Design review of the part built by this model. Coordinates are the model's own, in mm. A direction names the side the tool comes from. Round coordinates to 2 decimals unless told otherwise and drop trailing zeros. Order: outer loops, then holes, each group sorted by start corner. A loop starts at its lowest first (then second) coordinate and runs counter-clockwise, first axis right, second up. Notation, with made-up numbers: (74, 59.5) - (124, 59.5) arc R9 cw to (124, 67.5) - close; hole circle Ø9 at (23.5, 20). An arc over 180 degrees is marked (long way). Write item = value, one per line.
from build123d import *

# Parameters (mm, degrees)
F0_W     = 8.5
F0_H     = 2.5
F0_W_2   = 2
F0_H_2   = 1.512365222
F1_DEPTH = 19
F0_W_3   = 15
F0_H_3   = 9.5
F2_DEPTH = 8
F3_R     = 2
F4_SIZE2 = 1.4
F4_SIZE  = 3


with BuildPart() as f1:
    # F0 (on Top) → F1 (new body)
    with BuildSketch(Plane.XY):
        Polygon((-5.25, -2.25), (5.25, -2.25), (5.25, 2.25), (1, 2.25), (-1, 2.25), (-5.25, 2.25), align=None)
        Rectangle(F0_W, F0_H, mode=Mode.SUBTRACT)
        with Locations((0, 3.006182611)):
            Rectangle(F0_W_2, F0_H_2)
    extrude(amount=F1_DEPTH)

    # F0 (on Top) → F2 (join)
    with BuildSketch(Plane.XY):
        with Locations((0, 0.5852708127)):
            Rectangle(F0_W_3, F0_H_3)
        Polygon((5.25, 2.25), (5.25, -2.25), (-5.25, -2.25), (-5.25, 2.25), (-1, 2.25), (-1, 3.762365222), (1, 3.762365222), (1, 2.25), align=None, mode=Mode.SUBTRACT)
    extrude(amount=F2_DEPTH)

    # F3
    f3_edges = [f1.edges().sort_by_distance(p)[0] for p in [
        (-7.5, -4.164729, 4),
        (7.5, -4.164729, 4),
        (7.5, 5.335271, 4),
        (-7.5, 5.335271, 4),
    ]]
    fillet(f3_edges, radius=F3_R)

    # F4
    f4_edges = [f1.edges().sort_by_distance(p)[0] for p in [
        (0, 3.762365, 8),
    ]]
    f4_side = f1.faces().sort_by_distance((0, 3.762365, 13.5))[0]
    chamfer(f4_edges, length=F4_SIZE, length2=F4_SIZE2, reference=f4_side)


solid = f1.part
1) Clearance check with flat-ended pins moving along their axes: pin 1 Ø1.3 at (x, z) = (2.5, 14.5) entering from +Y; pin 2 Ø0.6 at (x, z) = (0.5, 14.5) entering from +Y; pin 3 Ø1.2 at (y, z) = (-0.5, 11) entering from -X. State where each tip first meets the part, or that it passes through.
Findings:
pin_1 = 2.25
pin_2 = 3.76
pin_3 = -5.25
2) We need section B-B on y = 0.5. Write out the cut boundary in (x, z), and give its area (3 significant figures).
Findings:
outline = (-7.5, 0) - (-4.25, 0) - (-4.25, 19) - (-5.25, 19) - (-5.25, 8) - (-7.5, 8) - close; (4.25, 0) - (7.5, 0) - (7.5, 8) - (5.25, 8) - (5.25, 19) - (4.25, 19) - close
area = 74.0 mm^2
3) We need section A-A on x = 2.5. Write out the cut boundary in (y, z), and give its area (3 significant figures).
Findings:
outline = (-4.16, 0) - (-1.25, 0) - (-1.25, 19) - (-2.25, 19) - (-2.25, 8) - (-4.16, 8) - close; (1.25, 0) - (5.34, 0) - (5.34, 8) - (2.25, 8) - (2.25, 19) - (1.25, 19) - close
area = 78.0 mm^2
4) We need section C-C on z = 6.5. Write out the cut boundary in (x, y), and give its area (3 significant figures).
Findings:
outline = (-7.5, -2.16) arc R2 ccw to (-5.5, -4.16) - (5.5, -4.16) arc R2 ccw to (7.5, -2.16) - (7.5, 3.34) arc R2 ccw to (5.5, 5.34) - (-5.5, 5.34) arc R2 ccw to (-7.5, 3.34) - close; hole (-4.25, -1.25) - (4.25, -1.25) - (4.25, 1.25) - (-4.25, 1.25) - close
area = 118 mm^2
5) We need section D-D on x = 0.5. Write out the cut boundary in (y, z), and give its area (3 significant figures).
Findings:
outline = (-4.16, 0) - (-1.25, 0) - (-1.25, 19) - (-2.25, 19) - (-2.25, 8) - (-4.16, 8) - close; (1.25, 0) - (5.34, 0) - (5.34, 8) - (5.16, 8) - (3.76, 11) - (3.76, 19) - (1.25, 19) - close
area = 96.7 mm^2
6) The part is to be moulded in two halves that separate along Y. For faces 5 (the flat face through (1, 3, 13)), 6 (the flat face through (0, 1.25, 9)), 7 (the flat face through (0, -2.25, 13)), 8 (the flat face through (-4.25, 0, 9)), say which applies: released by +Y, released by -Y, zero draft, split by the parting line, or undercut.
Findings:
face_5 = zero draft
face_6 = undercut
face_7 = released by -Y
face_8 = undercut
7) For faces 1 (the flat face through (0, 3.762, 15)), 2 (the flat face through (3, 2.25, 13)), 3 (the flat face through (-1, 3, 13)), 4 (the flat face through (-5.25, 0, 13)), list the 3-axis set-ups (+Z, -Z, +X, -X, +Y, -Y) from which the entire face can be reached by the end or side of a thin tool; tool diameter is ignored.
Findings:
face_1 = +Z, +X, -X, +Y
face_2 = +Z, +X, +Y
face_3 = +Z, -X, +Y
face_4 = +Z, -X, +Y, -Y
8) To check wall thickness, follow L1, parallel to Y at x = -3.25, z = 13; L2, parallel to X at y = -0.75, z = 18.25; L3, parallel to Y at x = 1, z = 6.75. State the ranges of each line that lie inside material, in increasing order. Write a range as from..to.
Findings:
L1 = -2.25..-1.25, 1.25..2.25
L2 = -5.25..-4.25, 4.25..5.25
L3 = -4.16..-1.25, 1.25..5.34
